```python
from build123d import *

# Parameters (mm, degrees)
EXTRUDE_1_DEPTH     = 80
SKETCH_2_W          = 28
SKETCH_2_H          = 76.722275626
CUT_EXTRUDE_2_DEPTH = 40
FILLET_1_R          = 1
FILLET_2_R          = 1
FILLET_3_R          = 1
SKETCH_4_W          = 17.86
SKETCH_4_H          = 9
EXTRUDE_2_DEPTH     = 10
EXTRUDE_3_DEPTH     = 17.89
SKETCH_6_R          = 2
CUT_EXTRUDE_3_DEPTH = 131.448569854


with BuildPart() as part:
    # 草图1 → 凸台-拉伸1 (new body)
    with BuildSketch(Plane.XY):
        with BuildLine():
            Line((0, 0), (0, 120))
            Line((0, 120), (2.5, 120))
            Line((2.5, 120), (2.5, 0))
            ThreePointArc((2.5, 0), (7.5, -5), (12.5, 0))
            Line((12.5, 0), (15, 0))
            ThreePointArc((15, 0), (7.5, -7.5), (0, 0))
        make_face()
    extrude(amount=EXTRUDE_1_DEPTH)

    # 草图2 → 切除-拉伸2 (cut, symmetric)
    with BuildSketch(Plane(origin=(2.5, 0, 0), x_dir=(0, 0, -1), z_dir=(1, 0, 0))):
        with Locations((-40, -7.5)):
            Rectangle(SKETCH_2_W, SKETCH_2_H)
    extrude(amount=CUT_EXTRUDE_2_DEPTH, both=True, mode=Mode.SUBTRACT)

    # 圆角1
    fillet_1_edges = [part.edges().sort_by_distance(p)[0] for p in [
        (12.5, 0, 67),
        (15, 0, 67),
        (12.5, 0, 13),
        (15, 0, 13),
    ]]
    fillet(fillet_1_edges, radius=FILLET_1_R)

    # 圆角2
    fillet_2_edges = [part.edges().sort_by_distance(p)[0] for p in [
        (0, 120, 40),
        (2.5, 120, 40),
    ]]
    fillet(fillet_2_edges, radius=FILLET_2_R)

    # 圆角3
    fillet_3_edges = [part.edges().sort_by_distance(p)[0] for p in [
        (0, 30.861137813, 40),
        (0, 15.430568906, 54),
        (0, 15.430568906, 26),
        (1.25, 30.861137813, 26),
        (2.5, 15.430568906, 26),
        (7.081868699, -4.982485947, 26),
        (2.5, 15.430568906, 54),
        (6.921352125, -7.477644458, 54),
        (1.25, 30.861137813, 54),
        (2.5, 30.861137813, 40),
        (13.669348036, 0, 26),
        (6.921352125, -7.477644458, 26),
        (14.682170815, -0.349556364, 26),
        (12.770582559, -0.236237384, 26),
        (7.081868699, -4.982485947, 54),
        (13.669348036, 0, 54),
        (14.682170815, -0.349556364, 54),
        (12.770582559, -0.236237384, 54),
    ]]
    fillet(fillet_3_edges, radius=FILLET_3_R)

    # 草图4 → 凸台-拉伸2 (add)
    with BuildSketch(Plane.ZY):
        with Locations((40, 64.861137813)):
            Rectangle(SKETCH_4_W, SKETCH_4_H)
    extrude(amount=EXTRUDE_2_DEPTH)

    # 草图5 → 凸台-拉伸3 (add)
    with BuildSketch(Plane.XY.offset(48.93)):
        with BuildLine():
            Line((-10, 69.361137813), (-10, 60.361137813))
            ThreePointArc((-10, 60.361137813), (-14.5, 64.861137813), (-10, 69.361137813))
        make_face()
    extrude(amount=-EXTRUDE_3_DEPTH)

    # 草图6 → 切除-拉伸3 (cut, through all)
    with BuildSketch(Plane.XY.offset(48.93)):
        with Locations((-10, 64.861137813)):
            Circle(SKETCH_6_R)
    extrude(amount=-CUT_EXTRUDE_3_DEPTH, mode=Mode.SUBTRACT)


solid = part.part
```
Part model, mm, in its own coordinate system. A direction names the side the tool comes from. Coordinates: 2 decimals unless noted, no trailing zeros. Write each loop counter-clockwise with the first axis right and the second up, starting at its lowest first coordinate (ties: lowest second). Pieces come first, ordered by that corner, then holes.
Item 1: Slice it at D-D (y = 35). Write the cut outline in (x, z), and give its area (3 significant figures).
Item 2: Slice it at C-C (x = -2). Write the cut outline in (y, z).
Item 3: Slice it at A-A (y = 21.5). Write the cut outline in (x, z), and give its area (3 significant figures).
Item 4: Pin check, flat tips, straight feed: pin 1 (1 mm diameter, centred on y = 71.5, z = 49, fed in from +X); pin 2 (1.5 mm diameter, centred on y = 84.5, z = 43.5, fed in from -X); pin 3 (1 mm diameter, centred on x = -11, z = 31.5, fed in from -Y). Stop position of each tip, or through.
Item 5: Mould opens along Z. For faces 1 (the face through (-7, 65, 48.93)), 2 (the face through (2.5, 60, 39)), 3 (the face through (1.3, 7.6, 26)), 4 (the face through (1.3, 7.6, 54)) say: released by +Z, released by -Z, zero draft, split by the parting line, or undercut.
Item 6: Which spindle directions (+Z, -Z, +X, -X, +Y, -Y) get a long thin tool onto all of the face, cutting with end or side? Do faces 5 (the face through (6.978, -4.973, 12.325)), 6 (the face through (7.08, -7.49, 67.32)), 7 (the face through (-5, 69.361, 40)), 8 (the face through (-5, 60.361, 40)), 9 (the face through (-12.2, 64.9, 31.04)). Say none if no direction does.
Item 7: Slice it at B-B (z = 44). Write the cut outline in (x, y), and give its area (3 significant figures).
Item 8: Probe line 1 (Y direction, x = -10, z = 42.75); line 2 (X direction, y = -1.5, z = 56.5); line 3 (X direction, y = 25.5, z = 56). List the from-to ranges inside material, lowest first.
Results found:
1. outline: (0, 0) - (2.5, 0) - (2.5, 80) - (0, 80) - close
1. area: 200 mm2
2. outline: (60.36, 31.07) - (69.36, 31.07) - (69.36, 48.93) - (60.36, 48.93) - close
3. outline: (0, 0) - (2.5, 0) - (2.5, 25) arc R1 ccw to (1.5, 26) - (1, 26) arc R1 ccw to (0, 25) - close; (0, 55) arc R1 ccw to (1, 54) - (1.5, 54) arc R1 ccw to (2.5, 55) - (2.5, 80) - (0, 80) - close
3. area: 129 mm2
4. pin 1: stops at x = 2.5
4. pin 2: stops at x = 0
4. pin 3: stops at y = 60.39
5. face 1: released by +Z
5. face 2: zero draft
5. face 3: undercut
5. face 4: undercut
6. face 5: +Z, -Z, +Y
6. face 6: +Z, -Z, -Y
6. face 7: +Z, -Z, -X, +Y
6. face 8: +Z, -Z, -X, -Y
6. face 9: -Z, -X, +Y, -Y
7. outline: (-10, 60.36) - (0, 60.36) - (0, 31.86) arc R1 ccw to (1, 30.86) - (1.5, 30.86) arc R1 ccw to (2.5, 31.86) - (2.5, 119) arc R1 ccw to (1.5, 120) - (1, 120) arc R1 ccw to (0, 119) - (0, 69.36) - (-10, 69.36) arc R4.5 ccw to start; hole circle Ø4 at (-10, 64.86)
7. area: 331 mm2
8. line 1: y = 60.36 to 62.86, 66.86 to 69.36
8. line 2: x = 0.15 to 2.73, 12.27 to 14.85
8. line 3: x = 0 to 2.5
